```python
from build123d import *

# Parameters (mm, degrees)
BOSS_EXTRUDE1_DEPTH = 50
CUT_EXTRUDE1_REACH  = 56.109
SKETCH2_R           = 1.5


with BuildPart() as part:
    # Sketch1 → Boss-Extrude1 (new body)
    with BuildSketch(Plane(origin=(0, 0, 0), x_dir=(1, 0, 0), z_dir=(0, 1, 0))):
        with BuildLine():
            Line((-15.1765625, 0), (15.1765625, 0))
            ThreePointArc((15.1765625, 0), (15.530115891, 0.146446609), (15.6765625, 0.5))
            Line((15.6765625, 0.5), (15.6765625, 12.99375))
            ThreePointArc((15.6765625, 12.99375), (15.530115891, 13.347303391), (15.1765625, 13.49375))
            Line((15.1765625, 13.49375), (10.025, 13.49375))
            ThreePointArc((10.025, 13.49375), (9.671446609, 13.347303391), (9.525, 12.99375))
            Line((9.525, 12.99375), (9.525, 7.64375))
            ThreePointArc((9.525, 7.64375), (9.671446609, 7.290196609), (10.025, 7.14375))
            Line((10.025, 7.14375), (11.2078125, 7.14375))
            ThreePointArc((11.2078125, 7.14375), (11.561365891, 6.997303391), (11.7078125, 6.64375))
            Line((11.7078125, 6.64375), (11.7078125, 4.071875))
            ThreePointArc((11.7078125, 4.071875), (11.561365891, 3.718321609), (11.2078125, 3.571875))
            Line((11.2078125, 3.571875), (-11.2078125, 3.571875))
            ThreePointArc((-11.2078125, 3.571875), (-11.561365891, 3.718321609), (-11.7078125, 4.071875))
            Line((-11.7078125, 4.071875), (-11.7078125, 6.64375))
            ThreePointArc((-11.7078125, 6.64375), (-11.561365891, 6.997303391), (-11.2078125, 7.14375))
            Line((-11.2078125, 7.14375), (-10.025, 7.14375))
            ThreePointArc((-10.025, 7.14375), (-9.671446609, 7.290196609), (-9.525, 7.64375))
            Line((-9.525, 7.64375), (-9.525, 12.99375))
            ThreePointArc((-9.525, 12.99375), (-9.671446609, 13.347303391), (-10.025, 13.49375))
            Line((-10.025, 13.49375), (-15.1765625, 13.49375))
            ThreePointArc((-15.1765625, 13.49375), (-15.530115891, 13.347303391), (-15.6765625, 12.99375))
            Line((-15.6765625, 12.99375), (-15.6765625, 0.5))
            ThreePointArc((-15.6765625, 0.5), (-15.530115891, 0.146446609), (-15.1765625, 0))
        make_face()
    extrude(amount=BOSS_EXTRUDE1_DEPTH)

    # Sketch2 → Cut-Extrude1 (cut, up to next)
    with BuildSketch(Plane.XY, mode=Mode.PRIVATE) as cut_extrude1_sk1:
        with Locations((0, 10)):
            Circle(SKETCH2_R)
    cut_extrude1_tool1 = extrude(cut_extrude1_sk1.sketch, amount=-CUT_EXTRUDE1_REACH, mode=Mode.PRIVATE) & part.part
    # Sketch2 → Cut-Extrude1 (cut, up to next)
    with BuildSketch(Plane.XY, mode=Mode.PRIVATE) as cut_extrude1_sk2:
        with Locations((0, 20)):
            Circle(SKETCH2_R)
    cut_extrude1_tool2 = extrude(cut_extrude1_sk2.sketch, amount=-CUT_EXTRUDE1_REACH, mode=Mode.PRIVATE) & part.part
    # Sketch2 → Cut-Extrude1 (cut, up to next)
    with BuildSketch(Plane.XY, mode=Mode.PRIVATE) as cut_extrude1_sk3:
        with Locations((0, 30)):
            Circle(SKETCH2_R)
    cut_extrude1_tool3 = extrude(cut_extrude1_sk3.sketch, amount=-CUT_EXTRUDE1_REACH, mode=Mode.PRIVATE) & part.part
    add(cut_extrude1_tool1.solids().sort_by_distance((0, 10, 0))[0], mode=Mode.SUBTRACT)
    add(cut_extrude1_tool2.solids().sort_by_distance((0, 20, 0))[0], mode=Mode.SUBTRACT)
    add(cut_extrude1_tool3.solids().sort_by_distance((0, 30, 0))[0], mode=Mode.SUBTRACT)


solid = part.part
```
Model file for the job. Use its own axes, mm. A direction names the side the tool comes from. Give positions to 0.01 mm unless a question says otherwise; leave off trailing zeros. Loops run counter-clockwise (first coordinate to the right, second up) from the corner with the lowest first, then second, coordinate; pieces in that order, holes last. Notation, with made-up numbers: (73.25, 66) -> (118.25, 66) arc R18 cw to (118.25, 85) -> close; hole circle Ø10 at (-4, 53.25). An arc over 180 degrees is marked (long way). Use CSV: the item, a comma, the result in double quotes. Start each with the question number.
1) Slice it at C-C on y = 47. Give the cut face in (x, z) (3 decimals).
2) Mould opens along X. For faces 1 (the flat face through (11.708, 25, -5)), 2 (the flat face through (-13, 25, -13.494)), 3 (the flat face through (-15.677, 25, -7)) say: released by +X, released by -X, zero draft, split by the parting line, or undercut.
3) Flat gauge pin, fed straight in: pin 1 Ø5 at (x, y) = (-3, 37.5) entering from -Z. Where does the tip first touch, or does it go through?
4) Slice it at B-B on z = -5.75. Give the cut face in (x, y), plus the area to 3 significant figures.
5) Tool access for faces 4 (the flat face through (-11, 25, -7.144)), 5 (the flat face through (9.525, 25, -10)), 6 (the cylindrical face through (-0.325, 8.536, -1.761)): list every direction of +Z, -Z, +X, -X, +Y, -Y with a clear straight run to the whole face (end or side of a thin tool).
6) Slice it at A-A on y = 30. Give the cut face in (x, z) (3 decimals).
7) Slice it at D-D on z = -11. Give the cut face in (x, y) (3 decimals), plus the area to 3 significant figures.
8) Wall check: line 1 (Y direction, x = 0, z = -1.65); line 2 (X direction, y = 47, z = -5); line 3 (Z direction, x = -11, y = 32). Give the ranges that are in metal, low to high.
Computed values:
1,outline,"(-15.677, -12.994) arc R0.5 ccw to (-15.177, -13.494) -> (-10.025, -13.494) arc R0.5 ccw to (-9.525, -12.994) -> (-9.525, -7.644) arc R0.5 ccw to (-10.025, -7.144) -> (-11.208, -7.144) arc R0.5 cw to (-11.708, -6.644) -> (-11.708, -4.072) arc R0.5 cw to (-11.208, -3.572) -> (11.208, -3.572) arc R0.5 cw to (11.708, -4.072) -> (11.708, -6.644) arc R0.5 cw to (11.208, -7.144) -> (10.025, -7.144) arc R0.5 ccw to (9.525, -7.644) -> (9.525, -12.994) arc R0.5 ccw to (10.025, -13.494) -> (15.177, -13.494) arc R0.5 ccw to (15.677, -12.994) -> (15.677, -0.5) arc R0.5 ccw to (15.177, 0) -> (-15.177, 0) arc R0.5 ccw to (-15.677, -0.5) -> close"
2,face 1,"undercut"
2,face 2,"zero draft"
2,face 3,"released by -X"
3,pin 1,"stops at z = -3.57"
4,outline,"(-15.68, 0) -> (-11.71, 0) -> (-11.71, 50) -> (-15.68, 50) -> close; (11.71, 0) -> (15.68, 0) -> (15.68, 50) -> (11.71, 50) -> close"
4,area,"397 mm^2"
5,face 4,"+Y, -Y"
5,face 5,"-Z, +Y, -Y"
5,face 6,"+Z, -Z"
6,outline,"(-15.677, -12.994) arc R0.5 ccw to (-15.177, -13.494) -> (-10.025, -13.494) arc R0.5 ccw to (-9.525, -12.994) -> (-9.525, -7.644) arc R0.5 ccw to (-10.025, -7.144) -> (-11.208, -7.144) arc R0.5 cw to (-11.708, -6.644) -> (-11.708, -4.072) arc R0.5 cw to (-11.208, -3.572) -> (-1.5, -3.572) -> (-1.5, 0) -> (-15.177, 0) arc R0.5 ccw to (-15.677, -0.5) -> close; (1.5, -3.572) -> (11.208, -3.572) arc R0.5 cw to (11.708, -4.072) -> (11.708, -6.644) arc R0.5 cw to (11.208, -7.144) -> (10.025, -7.144) arc R0.5 ccw to (9.525, -7.644) -> (9.525, -12.994) arc R0.5 ccw to (10.025, -13.494) -> (15.177, -13.494) arc R0.5 ccw to (15.677, -12.994) -> (15.677, -0.5) arc R0.5 ccw to (15.177, 0) -> (1.5, 0) -> close"
7,outline,"(-15.677, 0) -> (-9.525, 0) -> (-9.525, 50) -> (-15.677, 50) -> close; (9.525, 0) -> (15.677, 0) -> (15.677, 50) -> (9.525, 50) -> close"
7,area,"615 mm^2"
8,line 1,"y = 0 to 8.5, 11.5 to 18.5, 21.5 to 28.5, 31.5 to 50"
8,line 2,"x = -15.68 to -11.71, 11.71 to 15.68"
8,line 3,"z = -13.49 to -7.14, -3.57 to 0"
